```python
from build123d import *

# Parameters (mm, degrees)
F1_DEPTH = 20
F2_R     = 1.75
F3_DEPTH = 12.5
F4_R     = 5


with BuildPart() as f1:
    # F0 (on Top) → F1 (new body)
    with BuildSketch(Plane.XY):
        with BuildLine():
            Line((16.5, 10), (-16.5, 10))
            Line((-16.5, 10), (-16.5, -10))
            Line((-16.5, -10), (16.5, -10))
            Line((16.5, -10), (16.5, -5))
            Line((16.5, -5), (-6.5, -5))
            ThreePointArc((-6.5, -5), (-11.5, 0), (-6.5, 5))
            Line((-6.5, 5), (16.5, 5))
            Line((16.5, 5), (16.5, 10))
        make_face()
    extrude(amount=F1_DEPTH)

    # F2 (on Front) → F3 (cut, symmetric)
    with BuildSketch(Plane.XZ):
        with Locations((7.5, 15)):
            Circle(F2_R)
        with Locations((7.5, 5)):
            Circle(F2_R)
    extrude(amount=F3_DEPTH, both=True, mode=Mode.SUBTRACT)

    # F4
    f4_edges = [f1.edges().sort_by_distance(p)[0] for p in [
        (-16.5, 10, 10),
        (-16.5, -10, 10),
    ]]
    fillet(f4_edges, radius=F4_R)


solid = f1.part
```
Part model, mm, in its own coordinate system. A direction names the side the tool comes from. Coordinates: 2 decimals unless noted, no trailing zeros. Loops run counter-clockwise (first coordinate to the right, second up) from the corner with the lowest first, then second, coordinate; pieces in that order, holes last. Notation, with made-up numbers: (23.25, -14) - (31.25, -14) arc R18 ccw to (31.25, 15) - close; hole circle Ø4 at (3.5, 26). An arc over 180 degrees is marked (long way). Write item = value, one per line. Start each with the question number.
Item 1: Cut at B-B, the plane x = 6.5. Give the cut face in (y, z), and give its area (3 significant figures).
Item 2: 3-axis set-ups, long thin cutter, end or side, ignore diameter. For faces 1 (the flat face through (16.5, -8, 10)), 2 (the flat face through (5, -5, 10)): which of +Z, -Z, +X, -X, +Y, -Y reach the whole face in a straight line?
Item 3: Cut at D-D, the plane y = -7. Give the cut face in (x, z).
Item 4: Wall check: L1, parallel to Z at x = 7.5, y = -7.35; L2, parallel to Y at x = 9, z = 13.5; L3, parallel to X at y = -7.75, z = 14. Give the ranges that are in metal, low to high. Write a range as from..to.
Item 5: Cut at C-C, the plane x = -8. Give the cut face in (y, z).
Item 6: Flat gauge pins, fed straight in: pin 1 Ø1.5 at (x, y) = (3.5, 3.5) entering from +Z; pin 2 Ø1.5 at (y, z) = (-6, 11.5) entering from -X. Where does each tip first touch, or does it go through?
Item 7: Cut at A-A, the plane z = 5. Give the cut face in (x, y).
Item 8: Mould opens along Z. For faces 3 (the flat face through (-4, 7, 20)), 4 (the cylindrical face through (7.272, -7.465, 16.735)), 5 (the flat face through (2, -10, 10)) say: released by +Z, released by -Z, zero draft, split by the parting line, or undercut.
The answers:
q1.outline = (-10, 0) - (-5, 0) - (-5, 3.56) - (-10, 3.56) - close; (-10, 6.44) - (-5, 6.44) - (-5, 13.56) - (-10, 13.56) - close; (-10, 16.44) - (-5, 16.44) - (-5, 20) - (-10, 20) - close; (5, 0) - (10, 0) - (10, 3.56) - (5, 3.56) - close; (5, 6.44) - (10, 6.44) - (10, 13.56) - (5, 13.56) - close; (5, 16.44) - (10, 16.44) - (10, 20) - (5, 20) - close
q1.area = 143 mm2
q2.face_1 = +Z, -Z, +X, +Y, -Y
q2.face_2 = +Z, -Z, +X
q3.outline = (-16.08, 0) - (16.5, 0) - (16.5, 20) - (-16.08, 20) - close; hole circle Ø3.5 at (7.5, 5); hole circle Ø3.5 at (7.5, 15)
q4.L1 = 0..3.25, 6.75..13.25, 16.75..20
q4.L2 = -10..-5, 5..10
q4.L3 = -15.68..6.06, 8.94..16.5
q5.outline = (-10, 0) - (-4.77, 0) - (-4.77, 20) - (-10, 20) - close; (4.77, 0) - (10, 0) - (10, 20) - (4.77, 20) - close
q6.pin_1 = through
q6.pin_2 = -16.49
q7.outline = (-16.5, -5) arc R5 ccw to (-11.5, -10) - (5.75, -10) - (5.75, -5) - (-6.5, -5) arc R5 cw to (-6.5, 5) - (5.75, 5) - (5.75, 10) - (-11.5, 10) arc R5 ccw to (-16.5, 5) - close; (9.25, -10) - (16.5, -10) - (16.5, -5) - (9.25, -5) - close; (9.25, 5) - (16.5, 5) - (16.5, 10) - (9.25, 10) - close
q8.face_3 = released by +Z
q8.face_4 = undercut
q8.face_5 = zero draft
